Work out the finished part from the listing and answer in its coordinate system (mm). Round coordinates to 2 decimals unless told otherwise and drop trailing zeros. Loops run counter-clockwise (first coordinate to the right, second up) from the corner with the lowest first, then second, coordinate; pieces in that order, holes last. Notation, with made-up numbers: M 47,3 L 98,3 A25 cw 98,25 Z; hole C 48,24.5 d2. An arc over 180 degrees is marked long. One line per item, written item: value.
```python
from build123d import *

# Parameters (mm, degrees)
SKETCH1_W           = 57.1
SKETCH1_H           = 57.1
SKETCH1_R           = 2.15
SKETCH1_R_2         = 2.65
SKETCH1_R_3         = 5
BOSS_EXTRUDE1_DEPTH = 4.7625


with BuildPart() as part:
    # Sketch1 → Boss-Extrude1 (new body)
    with BuildSketch(Plane(origin=(0, 0, 0), x_dir=(1, 0, 0), z_dir=(0, 1, 0))):
        with Locations((28.55, 28.55)):
            Rectangle(SKETCH1_W, SKETCH1_H)
        with Locations(Location((12.993650814, 44.106349186, 0), (0, 0, 90))):
            Circle(SKETCH1_R, mode=Mode.SUBTRACT)
        with Locations(Location((12.993650814, 12.993650814, 0), (0, 0, 90))):
            Circle(SKETCH1_R, mode=Mode.SUBTRACT)
        with Locations(Location((44.106349186, 12.993650814, 0), (0, 0, 90))):
            Circle(SKETCH1_R, mode=Mode.SUBTRACT)
        with Locations(Location((44.106349186, 44.106349186, 0), (0, 0, 90))):
            Circle(SKETCH1_R, mode=Mode.SUBTRACT)
        with Locations(Location((5, 52.1, 0), (0, 0, 90))):
            Circle(SKETCH1_R_2, mode=Mode.SUBTRACT)
        with Locations(Location((52.1, 52.1, 0), (0, 0, 90))):
            Circle(SKETCH1_R_2, mode=Mode.SUBTRACT)
        with Locations(Location((52.1, 5, 0), (0, 0, 90))):
            Circle(SKETCH1_R_2, mode=Mode.SUBTRACT)
        with Locations(Location((5, 5, 0), (0, 0, 90))):
            Circle(SKETCH1_R_2, mode=Mode.SUBTRACT)
        with Locations(Location((28.55, 28.55, 0), (0, 0, 90))):
            Circle(SKETCH1_R_3, mode=Mode.SUBTRACT)
    extrude(amount=BOSS_EXTRUDE1_DEPTH)


solid = part.part
```
1) Find section B-B (x = 52.1). Give the vertices of the cut face in (y, z), then the cut area to 3 significant figures.
Check values:
outline: M 0,-57.1 L 4.76,-57.1 L 4.76,-54.75 L 0,-54.75 Z; M 0,-49.45 L 4.76,-49.45 L 4.76,-7.65 L 0,-7.65 Z; M 0,-2.35 L 4.76,-2.35 L 4.76,0 L 0,0 Z
area: 221 mm2
2) The mould has two halves that part along Z. Classify faces 1 (the face through (28, 2, -57.1)), 2 (the face through (51.304, 2.348, -7.528)), 3 (the face through (28, 2, 0)): +Z half, -Z half, draft (parallel to the pull), parting line (faces both ways), or undercut.
Check values:
face 1: -Z half
face 2: undercut
face 3: +Z half
3) Find section D-D (x = 28.55). Give the vertices of the cut face in (y, z).
Check values:
outline: M 0,-57.1 L 4.76,-57.1 L 4.76,-33.55 L 0,-33.55 Z; M 0,-23.55 L 4.76,-23.55 L 4.76,0 L 0,0 Z
4) This flat-tipped pin is pushed along its axis until it touches: pin 1 (4 mm diameter, centred on x = 44.11, z = -12.99, fed in from +Y). Where does it stop, or does it pass through?
Check values:
pin 1: through
5) Find section C-C (z = -28.55). Give the vertices of the cut face in (x, y).
Check values:
outline: M 0,0 L 23.55,0 L 23.55,4.76 L 0,4.76 Z; M 33.55,0 L 57.1,0 L 57.1,4.76 L 33.55,4.76 Z
6) Find section A-A (z = -13). Give the vertices of the cut face in (x, y).
Check values:
outline: M 0,0 L 10.84,0 L 10.84,4.76 L 0,4.76 Z; M 15.14,0 L 41.96,0 L 41.96,4.76 L 15.14,4.76 Z; M 46.26,0 L 57.1,0 L 57.1,4.76 L 46.26,4.76 Z
7) Find the intervals of material crossed by probe 1 along Z at (x, y) = (52.1, 2); probe 2 along X at (y, z) = (3, -52.1); probe 3 along Z at (x, y) = (50.5, 3.95), in increasing order. Write a range as from..to.
Check values:
probe 1: -57.1..-54.75, -49.45..-7.65, -2.35..0
probe 2: 0..2.35, 7.65..49.45, 54.75..57.1
probe 3: -57.1..-54.21, -49.99..-7.11, -2.89..0
